Solid Edge part; units mm, degrees
sketch "Sketch1" plane through (0, 0, 0) normal (0, 0, 1) x (1, 0, 0)
  line L0 (-80, -4.3375) -> (80, -4.3375)
  line L1 (80, -4.3375) -> (80, 10.6625)
  line L2 (80, 10.6625) -> (-80, 10.6625)
  line L3 (-80, 10.6625) -> (-80, -4.3375)
extrude "Protrusion1" add sketch "Sketch1" along normal blind 100
hole "Hole_1" at (0, -4.3375, 30) direction (0, 1, 0) diameter 4.917 end up to next thread major 6 thread length 2
hole "Hole_2" at (0, 3.1625, 100) direction (0, 0, -1) diameter 4.917 depth 12 thread major 6 thread length 2
hole "Hole_3" at (80, 3.1625, 77) direction (-1, 0, 0) diameter 4.917 depth 12 thread major 6 thread length 2
hole "Hole1" at (80, 4.1625, 23) direction (-1, 0, 0) diameter 4.917 depth 12 thread major 6 thread length 2
mirror "Mirror1" about plane through (0, 0, 0) normal (1, 0, 0) of "Hole_3", "Hole1"
Can you work these out from the model? Positions are in its coordinate system, mm. A direction names the side the tool comes from. Coordinates: 2 decimals unless noted, no trailing zeros. Loops run counter-clockwise (first coordinate to the right, second up) from the corner with the lowest first, then second, coordinate; pieces in that order, holes last. Notation, with made-up numbers: (11.25, -38) - (23.25, -38) arc R16 cw to (23.25, -30) - close; hole circle Ø9 at (-30, 86). An arc over 180 degrees is marked (long way). Put each result on its own line as item: value. Start each with the question number.
Item 1: Suppose I cut it at B-B (z = 30). Please give me the cut outline in (x, y), and give its area (3 significant figures).
Item 2: For pin 1 (1.5 mm diameter, centred on y = 2.5, z = 78, fed in from -X); pin 2 (3 mm diameter, centred on y = 4.16, z = 23, fed in from +X), each with a flat end and sliding along its axis, tell me the tip position at first contact or that it passes through.
Item 3: If we mould it in two halves opening along Y, with no side actions, what happens to faces 1 (the face through (1, 10.662, 49)), 2 (the face through (-68, 4, 23)), 3 (the face through (-80, 3, 49))? For each: +Y half, -Y half, draft (parallel to the pull), parting line (faces both ways), or undercut.
Item 4: Which directions (+Z, -Z, +X, -X, +Y, -Y) give clear straight access to the entire face, cutting with the end or side of a thin tool? Please do faces 4 (the face through (-73.916, 4.271, 25.456)), 5 (the face through (0.738, 3.057, 27.655)), 6 (the face through (-1, 7, 100)), 7 (the face through (0, 3, 88)), 8 (the face through (73.916, 4.054, 25.456)).
Item 5: Suppose I cut it at A-A (x = 0). Please give me the cut outline in (y, z).
Item 6: If I drill on line 1 along Y through (x, z) = (71.5, 23); line 2 along Y through (x, z) = (-70, 77); line 3 along X through (y, z) = (4.75, 30), over which ranges is the centre line in solid material (lowest first)?
Item 7: Suppose I cut it at C-C (z = 77). Please give me the cut outline in (x, y).
Here are the results:
1. outline: (-80, -4.34) - (-2.46, -4.34) - (-2.46, 10.66) - (-80, 10.66) - close; (2.46, -4.34) - (80, -4.34) - (80, 10.66) - (2.46, 10.66) - close
1. area: 2,330 mm²
2. pin 1: x = -68
2. pin 2: x = 68
3. face 1: +Y half
3. face 2: undercut
3. face 3: draft
4. face 4: -X
4. face 5: +Y, -Y
4. face 6: +Z, +X, -X, +Y, -Y
4. face 7: +Z
4. face 8: +X
5. outline: (-4.34, 0) - (10.66, 0) - (10.66, 27.54) - (-4.34, 27.54) - close; (-4.34, 32.46) - (10.66, 32.46) - (10.66, 100) - (5.62, 100) - (5.62, 88) - (0.7, 88) - (0.7, 100) - (-4.34, 100) - close
6. line 1: -4.34 to 1.7, 6.62 to 10.66
6. line 2: -4.34 to 0.7, 5.62 to 10.66
6. line 3: -80 to -2.46, 2.46 to 80
7. outline: (-80, -4.34) - (80, -4.34) - (80, 0.7) - (68, 0.7) - (68, 5.62) - (80, 5.62) - (80, 10.66) - (-80, 10.66) - (-80, 5.62) - (-68, 5.62) - (-68, 0.7) - (-80, 0.7) - close
